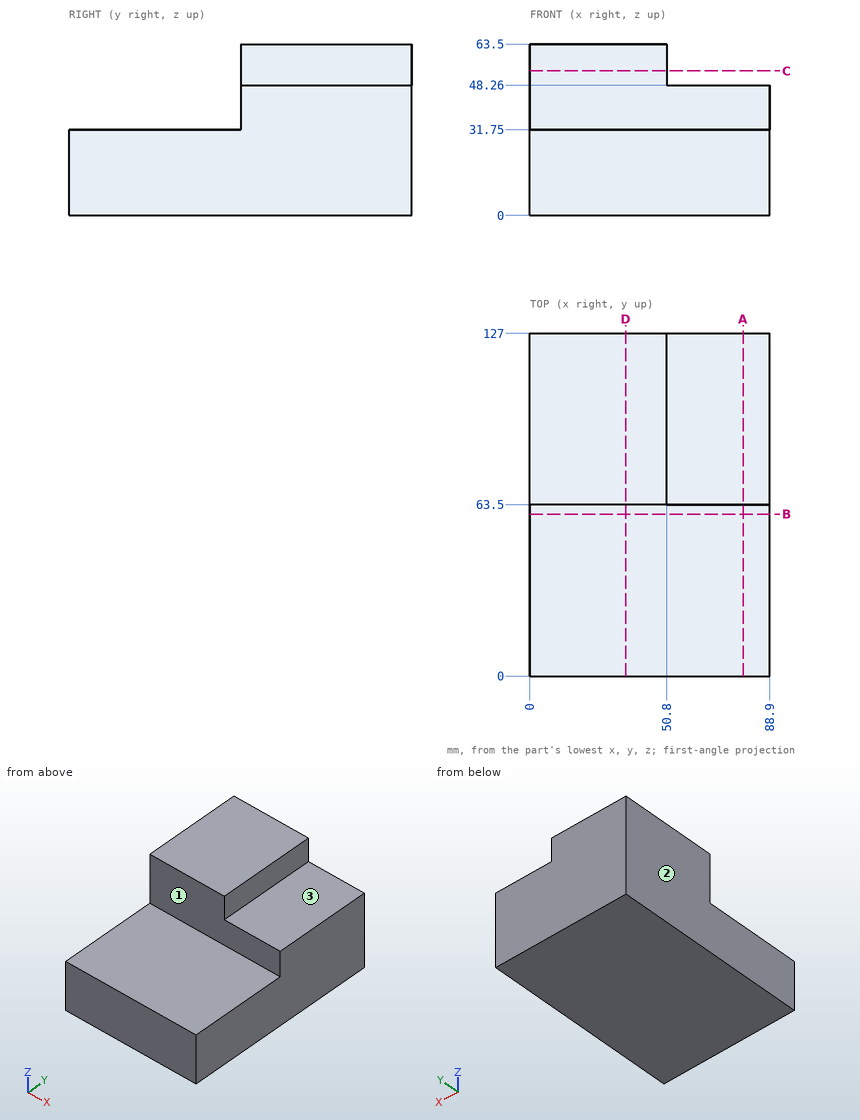
Design review of the part shown in the three views and the two pictorial views. Dimensions are in mm from the part's minimum x, y and z. A direction names the side the tool comes from. Coordinates: 2 decimals unless noted, no trailing zeros. Order: outer loops, then holes, each group sorted by start corner. A loop starts at its lowest first (then second) coordinate and runs counter-clockwise, first axis right, second up. Notation, with made-up numbers: (76, 49.5) -> (132, 49.5) arc R22 cw to (132, 80.5) -> close; hole circle Ø10 at (73, 61.25). An arc over 180 degrees is marked (long way). Use one line per item in the form item = value. Start each with the question number.
(1) For the marked faces 1, 2 and 3, list the 3-axis set-ups (+Z, -Z, +X, -X, +Y, -Y) from which the entire face can be reached by the end or side of a thin tool; tool diameter is ignored.
(2) Add section A-A on x = 79. State the section outline as (y, z) points.
(3) Add section C-C on z = 53.5. State the section outline as (x, y) points, plus the area to 3 significant figures.
(4) Add section B-B on y = 60. State the section outline as (x, z) points, plus the area to 3 significant figures.
(5) Insertion check: pin 1 (10 mm diameter, centred on y = 92, z = 53, fed in from -X); pin 2 (4.5 mm diameter, centred on y = 87, z = 55.5, fed in from +X); pin 3 (16 mm diameter, centred on x = 39.5, z = 43, fed in from -Y); pin 4 (4 mm diameter, centred on x = 58, y = 42, fed in from +Z). Each pin has a flat end and moves straight along its axis. Give the tip position at first contact, or say it passes through.
(6) For probe 1 along Z at (x, y) = (9.5, 38.5); probe 2 along X at (y, z) = (103, 51); probe 3 along Y at (x, z) = (59, 35), list the stretches that pass through material, from the lowest coordinate up.
(7) Add section D-D on x = 35.5. State the section outline as (y, z) points, plus the area to 3 significant figures.
Answer block:
q1.face_1 = +Z, +X, -X, -Y
q1.face_2 = +Z, -Z, -X, +Y, -Y
q1.face_3 = +Z, +X, +Y, -Y
q2.outline = (0, 0) -> (127, 0) -> (127, 48.26) -> (63.5, 48.26) -> (63.5, 31.75) -> (0, 31.75) -> close
q3.outline = (0, 63.5) -> (50.8, 63.5) -> (50.8, 127) -> (0, 127) -> close
q3.area = 3,230 mm²
q4.outline = (0, 0) -> (88.9, 0) -> (88.9, 31.75) -> (0, 31.75) -> close
q4.area = 2,820 mm²
q5.pin_1 = 0
q5.pin_2 = 50.8
q5.pin_3 = 63.5
q5.pin_4 = 31.75
q6.probe_1 = 0 to 31.75
q6.probe_2 = 0 to 50.8
q6.probe_3 = 63.5 to 127
q7.outline = (0, 0) -> (127, 0) -> (127, 63.5) -> (63.5, 63.5) -> (63.5, 31.75) -> (0, 31.75) -> close
q7.area = 6,050 mm²
